```python
from build123d import *

# Parameters (mm, degrees)
F0_W     = 38.4
F0_H     = 129.5
F0_W_2   = 31.4
F0_H_2   = 111
F1_DEPTH = 2
F2_DEPTH = 35
F3_SIZE2 = 17.5
F3_SIZE  = 7.5
F4_SIZE2 = 32.99999
F4_SIZE  = 5.99999
F6_DEPTH = 35.001
F7_W     = 32.5
F7_H     = 12.5
F8_DEPTH = 1
F9_SIZE2 = 10
F9_SIZE  = 1


# Not quite as in the source:
# - a fillet or chamfer is up to 0.001 mm smaller than in the source, because OpenCascade refuses the exact size


with BuildPart() as f1:
    # F0 (on Top) → F1 (new body)
    with BuildSketch(Plane.XY):
        with Locations((0, -5.75)):
            Rectangle(F0_W, F0_H)
        Rectangle(F0_W_2, F0_H_2, mode=Mode.SUBTRACT)
        Rectangle(F0_W_2, F0_H_2)
    extrude(amount=F1_DEPTH)

    # F0 (on Top) → F2 (join)
    with BuildSketch(Plane.XY):
        with Locations((0, -5.75)):
            Rectangle(F0_W, F0_H)
        Rectangle(F0_W_2, F0_H_2, mode=Mode.SUBTRACT)
    extrude(amount=F2_DEPTH)

    # F3
    f3_edges = [f1.edges().sort_by_distance(p)[0] for p in [
        (0, -70.5, 35),
    ]]
    f3_side = f1.faces().sort_by_distance((0, -69.149266, 35))[0]
    chamfer(f3_edges, length=F3_SIZE, length2=F3_SIZE2, reference=f3_side)

    # F4 (size 6 and 33 in the source; OpenCascade refuses exactly that, so slightly less here)
    f4_edges = [f1.edges().sort_by_distance(p)[0] for p in [
        (0, -55.5, 35),
    ]]
    f4_side = f1.faces().sort_by_distance((17.920994, -2, 35))[0]
    chamfer(f4_edges, length=F4_SIZE, length2=F4_SIZE2, reference=f4_side)

    # F5 (on face) → F6 (cut, through all)
    with BuildSketch(Plane.XY.offset(35)):
        Polygon((19.2, -28.5), (19.2, 17), (16.95, 19.25), (16.95, -30.75), align=None)
        Polygon((-19.2, 19.3914213562), (-16.95, 17.1414213562), (-16.95, 59), (-19.2, 59), align=None)
        Polygon((-16.95, -70.5), (-16.95, -28.6414213562), (-19.2, -30.8914213562), (-19.2, -70.5), align=None)
    extrude(amount=-F6_DEPTH, mode=Mode.SUBTRACT)

    # F7 (on face) → F8 (cut)
    with BuildSketch(Plane(origin=(0, -65.8965517241, 28.2413793103), x_dir=(1, 0, 0), z_dir=(0, -0.91914503, 0.3939192986))):
        with Locations((1.125, -2.1665561422)):
            Rectangle(F7_W, F7_H)
    extrude(amount=-F8_DEPTH, mode=Mode.SUBTRACT)

    # F9
    f9_edges = [f1.edges().sort_by_distance(p)[0] for p in [
        (0, 55.5, 2),
    ]]
    f9_side = f1.faces().sort_by_distance((0, 0, 2))[0]
    chamfer(f9_edges, length=F9_SIZE, length2=F9_SIZE2, reference=f9_side)


solid = f1.part
```
Part model, mm, in its own coordinate system. A direction names the side the tool comes from. Coordinates: 2 decimals unless noted, no trailing zeros. Order: outer loops, then holes, each group sorted by start corner. A loop starts at its lowest first (then second) coordinate and runs counter-clockwise, first axis right, second up. Notation, with made-up numbers: (49.5, 39) - (88.5, 39) arc R31 ccw to (88.5, 63) - close; hole circle Ø7 at (7.25, 54.25). An arc over 180 degrees is marked (long way). Return JSON: item names as keys, results as strings. Group by question number.
Item 1: Cut at C-C (y = -23). List the corners of the cut face in (x, z), plus the area to 3 significant figures.
Item 2: Drill centre lines: probe 1 along X at (y, z) = (-54, 26.5); probe 2 along X at (y, z) = (-8, 13); probe 3 along Z at (x, y) = (-15, 16.5). Where is each one in solid material? Low to high. Write a range as from..to.
Item 3: Which spindle directions (+Z, -Z, +X, -X, +Y, -Y) get a long thin tool onto all of the face, cutting with end or side? Do faces 1 (the face through (-15.7, -4, 18)), 2 (the face through (-3.1, -69.3, 20.3)). Say none if no direction does.
Item 4: Cut at B-B (z = 24). List the corners of the cut face in (x, y) (3 decimals).
Item 5: Cut at D-D (z = 29.5). List the corners of the cut face in (x, y) (3 decimals).
Item 6: Pull direction X, two halves, no side cores. Call faces 3 (the face through (19.2, 38, 17)), 4 (the face through (0, 55, 7)), 5 (the face through (0, -5, 0)): pulls with the +X half, pulls with the -X half, needs draft (parallel to the pull), parting line crosses it, or undercut.
Item 7: Pin check, flat tips, straight feed: pin 1 (6 mm diameter, centred on y = -0.5, z = 4.5, fed in from +X); pin 2 (4 mm diameter, centred on x = 7.5, y = -13, fed in from +Z); pin 3 (11.5 mm diameter, centred on x = -4.5, z = 25.5, fed in from -Y). Stop position of each tip, or through.
Check values:
{
 "1": {"outline": "(-19.2, 0) - (16.95, 0) - (16.95, 35) - (15.7, 35) - (15.7, 2) - (-15.7, 2) - (-15.7, 35) - (-19.2, 35) - close", "area": "229 mm2"},
 "2": {"probe 1": "x = -16.95..-15.7, 15.7..19.2", "probe 2": "x = -19.2..-15.7, 15.7..16.95", "probe 3": "z = 0..2"},
 "3": {"face 1": "+Z", "face 2": "+Z, +X, -X, -Y"},
 "4": {"outline": "(-19.2, -30.891) - (-16.95, -28.641) - (-16.95, -67.714) - (-15.125, -67.714) - (-15.125, -66.626) - (17.375, -66.626) - (17.375, -67.714) - (19.2, -67.714) - (19.2, -28.5) - (16.95, -30.75) - (16.95, 19.25) - (19.2, 17) - (19.2, 59) - (-16.95, 59) - (-16.95, 17.141) - (-19.2, 19.391) - close; hole (-15.7, -59.5) - (15.7, -59.5) - (15.7, 55.5) - (-15.7, 55.5) - close"},
 "5": {"outline": "(-19.2, -30.891) - (-16.95, -28.641) - (-16.95, -65.357) - (-15.125, -65.357) - (-15.125, -64.269) - (17.375, -64.269) - (17.375, -65.357) - (19.2, -65.357) - (19.2, -28.5) - (16.95, -30.75) - (16.95, 19.25) - (19.2, 17) - (19.2, 59) - (-16.95, 59) - (-16.95, 17.141) - (-19.2, 19.391) - close; hole (-15.7, -60.5) - (15.7, -60.5) - (15.7, 55.5) - (-15.7, 55.5) - close"},
 "6": {"face 3": "pulls with the +X half", "face 4": "undercut", "face 5": "needs draft"},
 "7": {"pin 1": "stops at x = 16.95", "pin 2": "stops at z = 2", "pin 3": "stops at y = -69.54"}
}
